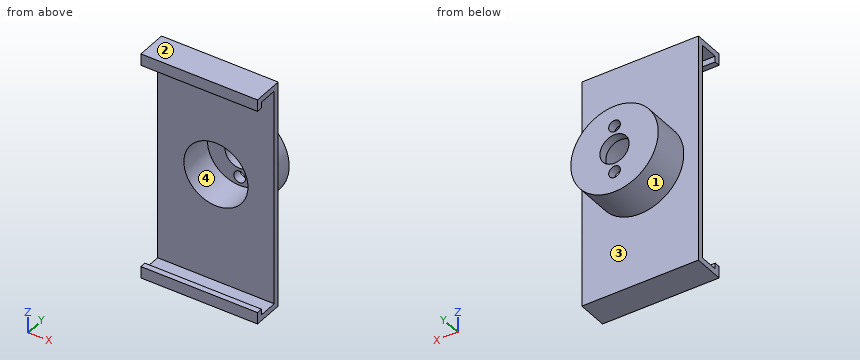
Autodesk Inventor part; units mm, degrees
ref_plane "YZ Plane" through (0, 0, 0) normal (1, 0, 0) x (0, 1, 0)
ref_plane "XZ Plane" through (0, 0, 0) normal (0, 1, 0) x (-1, 0, 0)
ref_plane "XY Plane" through (0, 0, 0) normal (0, 0, 1) x (1, 0, 0)
sketch "Boceto1" plane through (0, 0, 0) normal (0, 1, 0) x (-1, 0, 0)
  circle A0 centre (0, 0) radius 15
  circle A1 centre (0, 0) radius 5
  circle A2 centre (0, 8) radius 2
  circle A3 centre (0, -8) radius 2
  dimension "d0" = 30
  dimension "d1" = 10
  dimension "d2" = 4
  dimension "d3" = 8
  dimension "d4" = 4
  dimension "d5" = 8
extrude "Extrusión1" add sketch "Boceto1" against normal blind 3
sketch "Boceto2" plane through (0, -3, 0) normal (0, -1, 0) x (1, 0, 0)
  circle A0 centre (0, 0) radius 11
  circle A1 centre (0, 0) radius 15
  dimension "d8" = 22
extrude "Extrusión2" add sketch "Boceto2" along normal blind 10
sketch "Boceto5" plane through (0, 0, 0) normal (1, 0, 0) x (0, 1, 0)
  line L0 (-15, 0) -> (-15, 37.25)
  line L1 (-32.5779, 0) -> (6.5779, 0) construction
  line L2 (-13, 39.25) -> (-13, 0)
  line L3 (-13, 39.25) -> (-23.5, 39.25)
  line L4 (-23.5, 39.25) -> (-23.5, 35.25)
  line L5 (-23.5, 35.25) -> (-21.5, 35.25)
  line L6 (-21.5, 35.25) -> (-21.5, 37.25)
  line L7 (-21.5, 37.25) -> (-15, 37.25)
  line L8 (-15, 0) -> (-15, -37.25)
  line L9 (-13, -39.25) -> (-13, 0)
  line L10 (-13, -39.25) -> (-23.5, -39.25)
  line L11 (-23.5, -39.25) -> (-23.5, -35.25)
  line L12 (-23.5, -35.25) -> (-21.5, -35.25)
  line L13 (-21.5, -35.25) -> (-21.5, -37.25)
  line L14 (-21.5, -37.25) -> (-15, -37.25)
  point P0 (0, 0)
  dimension "d27" = 10.5
  dimension "d28" = 4
  dimension "d29" = 2
  dimension "d30" = 2
extrude "Extrusión5" add sketch "Boceto5" along normal mid plane 40
sketch "Boceto6" plane through (0, -13, 0) normal (0, 1, 0) x (1, 0, 0)
  circle A0 centre (0, 0) radius 11
  point P0 (0, 0)
extrude "Extrusión6" cut sketch "Boceto6" against normal through all
properties part number "motor_prueba_3DPrint"
Can you work these out from the model? Positions are in its coordinate system, mm. Face numbers are marked on the shaded views. A direction names the side the tool comes from. Coordinates: 2 decimals unless noted, no trailing zeros. Write each loop counter-clockwise with the first axis right and the second up, starting at its lowest first coordinate (ties: lowest second). Pieces come first, ordered by that corner, then holes. Notation, with made-up numbers: (2.5, 48.5) - (40.5, 48.5) arc R21 ccw to (40.5, 76.5) - close; hole circle Ø8 at (68, -24.75). An arc over 180 degrees is marked (long way). Return JSON: item names as keys, results as strings.
Q1. If we section it at C-C (x = 0): Count the separate pieces of the cut face and the enclosed holes in it, then the cut area to 3 significant figures.
Computed values:
{"separate pieces": "4", "enclosed holes": "0", "area": "271 mm2"}
Q2. If we section it at A-A (y = -19.25): Please give me the cut outline in (x, z).
Computed values:
{"outline": "(-20, -39.25) - (20, -39.25) - (20, -37.25) - (-20, -37.25) - close; (-20, 37.25) - (20, 37.25) - (20, 39.25) - (-20, 39.25) - close"}
Q3. If we section it at D-D (x = 8): Please give me the cut outline in (y, z), then the cut area to 3 significant figures.
Computed values:
{"outline": "(-23.5, -39.25) - (-13, -39.25) - (-13, -12.69) - (0, -12.69) - (0, 12.69) - (-13, 12.69) - (-13, 39.25) - (-23.5, 39.25) - (-23.5, 35.25) - (-21.5, 35.25) - (-21.5, 37.25) - (-15, 37.25) - (-15, 7.55) - (-3, 7.55) - (-3, -7.55) - (-15, -7.55) - (-15, -37.25) - (-21.5, -37.25) - (-21.5, -35.25) - (-23.5, -35.25) - close", "area": "348 mm2"}
Q4. Please list where these lines run through material, in increasing order: L1, parallel to Z at x = 0, y = -1.9; L2, parallel to Z at x = -8.5, y = -19; L3, parallel to Z at x = 0, y = -6. Write a range as from..to.
Computed values:
{"L1": "z = -15..-10, -6..-5, 5..6, 10..15", "L2": "z = -39.25..-37.25, 37.25..39.25", "L3": "z = -15..-11, 11..15"}
Q5. On a 3-axis mill with a long thin cutter (end or side, diameter ignored), from which of +Z, -Z, +X, -X, +Y, -Y can I reach the whole of each face in a straight line? I mean the marked faces 1 and 2. Say none if no direction works.
Computed values:
{"face 1": "+Y", "face 2": "+Z, +X, -X, +Y, -Y"}
Q6. If we section it at B-B (z = 0): Please give me the cut outline in (x, y).
Computed values:
{"outline": "(-20, -15) - (-11, -15) - (-11, -3) - (-5, -3) - (-5, 0) - (-15, 0) - (-15, -13) - (-20, -13) - close; (5, -3) - (11, -3) - (11, -15) - (20, -15) - (20, -13) - (15, -13) - (15, 0) - (5, 0) - close"}
Q7. Thinking about a two-plate mould opening in Y: for the marked faces 3 and 4, which applies, +Y half, -Y half, draft (parallel to the pull), parting line (faces both ways), or undercut?
Computed values:
{"face 3": "+Y half", "face 4": "draft"}
Q8. I'm going to push flat-ended pins straight in: pin 1 Ø6 at (x, z) = (-6.5, -24) entering from +Y; pin 2 Ø8 at (y, z) = (-8.5, 8) entering from +X; pin 3 Ø24 at (x, z) = (2, 2.5) entering from -Y. Where does each tip first touch, or does it pass through?
Computed values:
{"pin 1": "stops at y = -13", "pin 2": "stops at x = 14.46", "pin 3": "stops at y = -15"}
